The listing builds one solid part. Answer for the finished solid, in the listing's coordinates (mm). Face numbers are marked on the shaded views. A direction names the side the tool comes from. Coordinates: 2 decimals unless noted, no trailing zeros. Order: outer loops, then holes, each group sorted by start corner. A loop starts at its lowest first (then second) coordinate and runs counter-clockwise, first axis right, second up. Notation, with made-up numbers: M 30,52 L 56,52 A14 ccw 56,73 Z; hole C 42,50.25 d2. An arc over 180 degrees is marked long. One line per item, written item: value. Start each with the question number.
Q1. Each of these flat-tipped pins is pushed along its axis until it touches: pin 1 Ø12 at (x, y) = (-49, -0.5) entering from -Z; pin 2 Ø2 at (x, z) = (-7.5, -1.5) entering from -Y. Where does it stop, or does it pass through?
Q2. For the marked faces 1 and 2, determine the directions among +Z, -Z, +X, -X, +Y, -Y from which every point of the face is accessible in a straight line to the end or side of a thin tool.
Q3. The part is cut by section D-D on y = 27.5. Give the vertices of the cut face in (x, z).
Q4. Straight lines are drawn through the part: line 1 along X through (y, z) = (-5, -0.6) (3 decimals); line 2 along Y through (x, z) = (-32, -0.3); line 3 along X through (y, z) = (13.5, -0.5) (3 decimals). For each, find the intervals that lie inside material, in ascending order. Write a range as [from, to].
Q5. The part is cut by section B-B on x = -53. Give the vertices of the cut face in (y, z), then the cut area to 3 significant figures.
Q6. The part is cut by section A-A on x = 18. Give the vertices of the cut face in (y, z).
Q7. The part is cut by section C-C on z = -1.85. Give the vertices of the cut face in (x, y), then the cut area to 3 significant figures.
```python
from build123d import *

# Parameters (mm, degrees)
F1_DEPTH      = 63.5
F1_DEPTH_BACK = 63.5
F3_DEPTH      = 3.6078
F5_DEPTH      = 3.6078


with BuildPart() as f1:
    # F0 (on Right) → F1 (new body, two sides)
    with BuildSketch(Plane.YZ) as f1_sk:
        Polygon((-31.75, -0.9017), (29.9466, -0.9017), (29.9466, -2.7051), (31.75, -2.7051), (31.75, -0.9017), (31.75, 0.9017), (-31.75, 0.9017), align=None)
    extrude(amount=F1_DEPTH)
    extrude(f1_sk.sketch, amount=-F1_DEPTH_BACK)

    # F2 (on face) → F3 (cut, through all)
    with BuildSketch(Plane.XY.offset(0.9017)):
        with BuildLine():
            Line((-25.4, 17.0434), (-34.925, 17.0434))
            ThreePointArc((-34.925, 17.0434), (-37.170064, 16.113464), (-38.1, 13.8684))
            ThreePointArc((-38.1, 13.8684), (-37.170064, 11.623336), (-34.925, 10.6934))
            Line((-34.925, 10.6934), (-28.575, 10.6934))
            Line((-28.575, 10.6934), (-28.575, 4.3434))
            Line((-28.575, 4.3434), (-34.925, 4.3434))
            ThreePointArc((-34.925, 4.3434), (-37.170064, 3.413464), (-38.1, 1.1684))
            ThreePointArc((-38.1, 1.1684), (-37.170064, -1.076664), (-34.925, -2.0066))
            Line((-34.925, -2.0066), (-28.575, -2.0066))
            Line((-28.575, -2.0066), (-28.575, -8.3566))
            Line((-28.575, -8.3566), (-34.925, -8.3566))
            ThreePointArc((-34.925, -8.3566), (-37.170064, -9.286536), (-38.1, -11.5316))
            ThreePointArc((-38.1, -11.5316), (-37.170064, -13.776664), (-34.925, -14.7066))
            Line((-34.925, -14.7066), (-25.4, -14.7066))
            ThreePointArc((-25.4, -14.7066), (-23.154936, -13.776664), (-22.225, -11.5316))
            Line((-22.225, -11.5316), (-22.225, -8.3566))
            Line((-22.225, -8.3566), (-15.875, -8.3566))
            ThreePointArc((-15.875, -8.3566), (-13.629936, -7.426664), (-12.7, -5.1816))
            ThreePointArc((-12.7, -5.1816), (-13.629936, -2.936536), (-15.875, -2.0066))
            Line((-15.875, -2.0066), (-22.225, -2.0066))
            Line((-22.225, -2.0066), (-22.225, 4.3434))
            Line((-22.225, 4.3434), (-15.875, 4.3434))
            ThreePointArc((-15.875, 4.3434), (-13.629936, 5.273336), (-12.7, 7.5184))
            ThreePointArc((-12.7, 7.5184), (-13.629936, 9.763464), (-15.875, 10.6934))
            Line((-15.875, 10.6934), (-22.225, 10.6934))
            Line((-22.225, 10.6934), (-22.225, 13.8684))
            ThreePointArc((-22.225, 13.8684), (-23.154936, 16.113464), (-25.4, 17.0434))
        make_face()
    extrude(amount=-F3_DEPTH, mode=Mode.SUBTRACT)

    # F4 (on face) → F5 (cut, through all)
    with BuildSketch(Plane.XY.offset(0.9017)):
        with BuildLine():
            Line((25.4, 17.0434), (15.875, 17.0434))
            ThreePointArc((15.875, 17.0434), (13.629936, 16.113464), (12.7, 13.8684))
            ThreePointArc((12.7, 13.8684), (13.629936, 11.623336), (15.875, 10.6934))
            Line((15.875, 10.6934), (22.225, 10.6934))
            Line((22.225, 10.6934), (22.225, 4.3434))
            Line((22.225, 4.3434), (15.875, 4.3434))
            ThreePointArc((15.875, 4.3434), (13.629936, 3.413464), (12.7, 1.1684))
            ThreePointArc((12.7, 1.1684), (13.629936, -1.076664), (15.875, -2.0066))
            Line((15.875, -2.0066), (22.225, -2.0066))
            Line((22.225, -2.0066), (22.225, -8.3566))
            Line((22.225, -8.3566), (15.875, -8.3566))
            ThreePointArc((15.875, -8.3566), (13.629936, -9.286536), (12.7, -11.5316))
            ThreePointArc((12.7, -11.5316), (13.629936, -13.776664), (15.875, -14.7066))
            Line((15.875, -14.7066), (25.4, -14.7066))
            ThreePointArc((25.4, -14.7066), (27.645064, -13.776664), (28.575, -11.5316))
            Line((28.575, -11.5316), (28.575, -8.3566))
            Line((28.575, -8.3566), (34.925, -8.3566))
            ThreePointArc((34.925, -8.3566), (37.170064, -7.426664), (38.1, -5.1816))
            ThreePointArc((38.1, -5.1816), (37.170064, -2.936536), (34.925, -2.0066))
            Line((34.925, -2.0066), (28.575, -2.0066))
            Line((28.575, -2.0066), (28.575, 4.3434))
            Line((28.575, 4.3434), (34.925, 4.3434))
            ThreePointArc((34.925, 4.3434), (37.170064, 5.273336), (38.1, 7.5184))
            ThreePointArc((38.1, 7.5184), (37.170064, 9.763464), (34.925, 10.6934))
            Line((34.925, 10.6934), (28.575, 10.6934))
            Line((28.575, 10.6934), (28.575, 13.8684))
            ThreePointArc((28.575, 13.8684), (27.645064, 16.113464), (25.4, 17.0434))
        make_face()
    extrude(amount=-F5_DEPTH, mode=Mode.SUBTRACT)


solid = f1.part
```
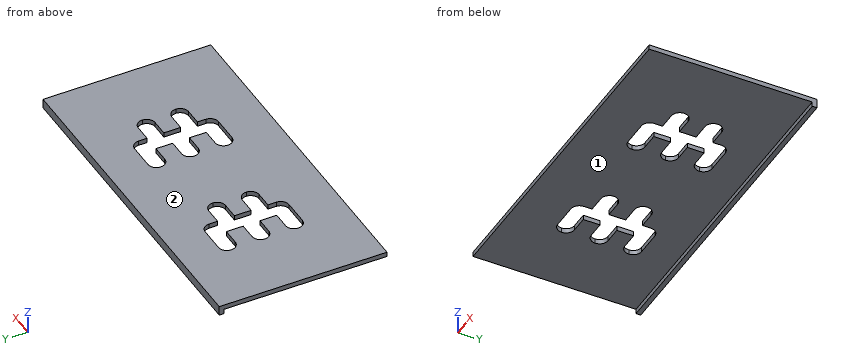
Output:
1. pin 1: stops at z = -0.9
1. pin 2: stops at y = -31.75
2. face 1: -Z, +X, -X, -Y
2. face 2: +Z, +X, -X, +Y, -Y
3. outline: M -63.5,-0.9 L 63.5,-0.9 L 63.5,0.9 L -63.5,0.9 Z
4. line 1: x = [-63.5, -28.575], [-12.705, 22.225], [38.095, 63.5]
4. line 2: y = [-31.75, -14.71], [-8.36, -2.01], [4.34, 10.69], [17.04, 31.75]
4. line 3: x = [-63.5, -38.079], [-22.225, 12.721], [28.575, 63.5]
5. outline: M -31.75,-0.9 L 29.95,-0.9 L 29.95,-2.71 L 31.75,-2.71 L 31.75,0.9 L -31.75,0.9 Z
5. area: 118 mm^2
6. outline: M -31.75,-0.9 L -14.71,-0.9 L -14.71,0.9 L -31.75,0.9 Z; M -8.36,-0.9 L -2.01,-0.9 L -2.01,0.9 L -8.36,0.9 Z; M 4.34,-0.9 L 10.69,-0.9 L 10.69,0.9 L 4.34,0.9 Z; M 17.04,-0.9 L 29.95,-0.9 L 29.95,-2.71 L 31.75,-2.71 L 31.75,0.9 L 17.04,0.9 Z
7. outline: M -63.5,29.95 L 63.5,29.95 L 63.5,31.75 L -63.5,31.75 Z
7. area: 229 mm^2
